Source: CAD feature listing. Evaluate the final solid. Frame: model axes, mm. A direction names the side the tool comes from. Round coordinates to 2 decimals unless told otherwise and drop trailing zeros. Loops run counter-clockwise (first coordinate to the right, second up) from the corner with the lowest first, then second, coordinate; pieces in that order, holes last.
Item 1: Section query A-A on x = 0. Return loops of the section in (y, z).
Item 2: Pull-direction query (Z, two-part tool) for faces 3 (the flat face through (-4.5, 0.1, 0)), 4 (the flat face through (-4.5, 0.1, 95)), 5 (the flat face through (0, 4, 47)), 6 (the cylindrical face through (-4.49, 0.35, 6.56)); classes: released by +Z, released by -Z, zero draft, split by the parting line, or undercut.
Item 3: Section query B-B on y = 3. Return loops of the section in (x, z).
Item 4: Section query C-C on z = 40.5. Return loops of the section in (x, y), then the cut area to 3 significant figures.
Item 5: Ray query, L1, parallel to Z at x = 0, y = -4.3; L2, parallel to Y at x = -3.5, z = 30. Return the intervals inside material, ascending.
Item 6: Access query for faces 1 (the flat face through (-4, 0, 47)), 2 (the flat face through (0, 5, 47)). Directions: +Z, -Z, +X, -X, +Y, -Y. A direction counts if a zero-diameter tool reaches every point of the face in a straight line with its end or side. Return the directions, or none.
Item 7: First-contact query: P1, Ø3, axis at y = 0, z = 5, coming from the -X side. Flat tip, straight axial feed; report the tip coordinate or a pass-through.
```python
from build123d import *

# Parameters (mm, degrees)
SKETCH_1_W          = 10
SKETCH_1_H          = 10
SKETCH_1_W_2        = 8
SKETCH_1_H_2        = 8
EXTRUDE_1_DEPTH     = 95
SKETCH_3_R          = 1.6
CUT_EXTRUDE_2_DEPTH = 96.655632349
SKETCH_4_R          = 1.6
CUT_EXTRUDE_3_DEPTH = 96.655632349


with BuildPart() as part:
    # ｽｹｯﾁ1 → 押し出し-薄板1 (new body)
    with BuildSketch(Plane.XY):
        Rectangle(SKETCH_1_W, SKETCH_1_H)
        Rectangle(SKETCH_1_W_2, SKETCH_1_H_2, mode=Mode.SUBTRACT)
    extrude(amount=EXTRUDE_1_DEPTH)

    # ｽｹｯﾁ3 → ｶｯﾄ - 押し出し2 (cut, through all)
    with BuildSketch(Plane(origin=(0, 5, 0), x_dir=(1, 0, 0), z_dir=(0, 1, 0))):
        with Locations(Location((0, -56.5, 0), (0, 0, 180))):
            Circle(SKETCH_3_R)
        with Locations(Location((0, -36.5, 0), (0, 0, 180))):
            Circle(SKETCH_3_R)
    extrude(amount=-CUT_EXTRUDE_2_DEPTH, mode=Mode.SUBTRACT)

    # ｽｹｯﾁ4 → ｶｯﾄ - 押し出し3 (cut, through all)
    with BuildSketch(Plane(origin=(5, 0, 0), x_dir=(0, 0, -1), z_dir=(1, 0, 0))):
        with Locations(Location((-90, 0, 0), (0, 0, 90))):
            Circle(SKETCH_4_R)
        with Locations(Location((-5, 0, 0), (0, 0, 270))):
            Circle(SKETCH_4_R)
    extrude(amount=-CUT_EXTRUDE_3_DEPTH, mode=Mode.SUBTRACT)


solid = part.part
```
Data:
1. outline: (-5, 0) - (-4, 0) - (-4, 34.9) - (-5, 34.9) - close; (-5, 38.1) - (-4, 38.1) - (-4, 54.9) - (-5, 54.9) - close; (-5, 58.1) - (-4, 58.1) - (-4, 95) - (-5, 95) - close; (4, 0) - (5, 0) - (5, 34.9) - (4, 34.9) - close; (4, 38.1) - (5, 38.1) - (5, 54.9) - (4, 54.9) - close; (4, 58.1) - (5, 58.1) - (5, 95) - (4, 95) - close
2. face 3: released by -Z
2. face 4: released by +Z
2. face 5: zero draft
2. face 6: undercut
3. outline: (-5, 0) - (-4, 0) - (-4, 95) - (-5, 95) - close; (4, 0) - (5, 0) - (5, 95) - (4, 95) - close
4. outline: (-5, -5) - (5, -5) - (5, 5) - (-5, 5) - close; hole (-4, -4) - (4, -4) - (4, 4) - (-4, 4) - close
4. area: 36.0 mm2
5. L1: z = 0 to 34.9, 38.1 to 54.9, 58.1 to 95
5. L2: y = -5 to -4, 4 to 5
6. face 1: +Z, -Z
6. face 2: +Z, -Z, +X, -X, +Y
7. P1: passes through
